Check sheet for the modelled part. Datum: model origin and axes. Units: mm. A direction names the side the tool comes from. Give positions to 0.01 mm unless a question says otherwise; leave off trailing zeros. Write each loop counter-clockwise with the first axis right and the second up, starting at its lowest first coordinate (ties: lowest second). Pieces come first, ordered by that corner, then holes. Notation, with made-up numbers: (36.5, 2) -> (43.5, 2) arc R16 ccw to (43.5, 12) -> close; hole circle Ø3 at (-26.5, 59). An arc over 180 degrees is marked (long way). Return JSON: item names as keys, results as strings.
from build123d import *
from build123d.topology import SkipClean

# Parameters (mm, degrees)
BASE_FLANGE1_DEPTH       = 2.54
SKETCHED_START           = 383.54
SKETCHED_BEND2_OUTLINE_W = 2.54
SKETCHED_BEND2_OUTLINE_H = 495.3
SKETCHED_BEND2_DEPTH     = 378.46
SKETCHED_START_2         = 381
SKETCHED_BEND2_2_DEPTH   = 2.221317884
SKETCHED_START_3         = 380.2634
SKETCHED_BEND2_3_DEPTH   = 3.2766
SKETCHED_START_4         = -438.15
SKETCHED_BEND2_4_DEPTH   = 495.3
SKETCHED_START_5         = 2.131240091
SKETCHED_BEND7_DEPTH     = 25
SKETCHED_BEND7_2_DEPTH   = 12.3
SKETCHED_START_6         = -384.2766
SKETCHED_BEND7_3_DEPTH   = 3.158240169
SKETCHED_START_7         = 0.118359831
SKETCHED_BEND7_4_DEPTH   = 3.158240169
SKETCHED_START_8         = 14.431240091
SKETCHED_BEND7_5_DEPTH   = 12.7
SKETCHED_BEND7_6_DEPTH   = 12.7
SKETCH20_R               = 8
CUT_EXTRUDE1_DEPTH       = 665.217598099
SKETCH21_R               = 12.7
CUT_EXTRUDE2_DEPTH       = 2.54
CUT_EXTRUDE3_DEPTH       = 2.54


with BuildPart() as part:
    # Base-Flange1: sheet metal written as solids
    # Sketch1 → Base-Flange1 (new body)
    with BuildSketch(Plane(origin=(0, 0, 0), x_dir=(1, 0, 0), z_dir=(0, 1, 0))):
        with BuildLine():
            Line((0, 0), (0, 381))
            Line((0, 381), (384.81, 381))
            Line((384.81, 381), (384.81, 438.15))
            Line((384.81, 438.15), (397.11, 438.15))
            ThreePointArc((397.11, 438.15), (406.090256121, 434.430256121), (409.81, 425.45))
            Line((409.81, 425.45), (409.81, 381))
            Line((409.81, 381), (690.157951031, 381))
            Line((690.157951031, 381), (762, 381))
            Line((762, 381), (762, 0.361010763))
            Line((762, 0.361010763), (690.158858088, 0))
            Line((690.158858088, 0), (409.81, 0))
            Line((409.81, 0), (409.81, -44.45))
            ThreePointArc((409.81, -44.45), (406.090256121, -53.430256121), (397.11, -57.15))
            Line((397.11, -57.15), (384.81, -57.15))
            Line((384.81, -57.15), (384.81, 0))
            Line((384.81, 0), (0, 0))
        make_face()
    extrude(amount=-BASE_FLANGE1_DEPTH)

    # Sketched Bend2: read off the stored shape, not the designer's step
    # Sketched Bend2 outline → Sketched Bend2 (cut)
    with BuildSketch(Plane.YZ.offset(SKETCHED_START)):
        with Locations((-1.27, -190.5)):
            Rectangle(SKETCHED_BEND2_OUTLINE_W, SKETCHED_BEND2_OUTLINE_H)
    extrude(amount=SKETCHED_BEND2_DEPTH, mode=Mode.SUBTRACT)

    # Sketched Bend2 2 outline → Sketched Bend2 2 (add)
    with BuildSketch(Plane.YZ.offset(SKETCHED_START_2)):
        with BuildLine():
            Line((2.131240091, 57.15), (2.131240091, 0))
            Line((2.131240091, 0), (0, 0))
            Line((0, 0), (0, -381))
            Line((0, -381), (2.131240091, -381))
            Line((2.131240091, -381), (2.131240091, -438.15))
            Line((2.131240091, -438.15), (14.431240091, -438.15))
            ThreePointArc((14.431240091, -438.15), (23.411496212, -434.430256121), (27.131240091, -425.45))
            Line((27.131240091, -425.45), (27.131240091, -381))
            Line((27.131240091, -381), (379.321240091, -381))
            Line((379.321240091, -381), (379.321240091, -0.361010763))
            Line((379.321240091, -0.361010763), (307.480098179, 0))
            Line((307.480098179, 0), (27.131240091, 0))
            Line((27.131240091, 0), (27.131240091, 44.45))
            ThreePointArc((27.131240091, 44.45), (23.411496212, 53.430256121), (14.431240091, 57.15))
            Line((14.431240091, 57.15), (2.131240091, 57.15))
        make_face()
    extrude(amount=SKETCHED_BEND2_2_DEPTH)

    # Sketched Bend2 3 outline → Sketched Bend2 3 (add)
    with BuildSketch(Plane.YZ.offset(SKETCHED_START_3)):
        with BuildLine():
            Line((2.131240091, 57.15), (2.131240091, 0))
            Line((2.131240091, 0), (0, 0))
            Line((0, 0), (0, -381))
            Line((0, -381), (2.131240091, -381))
            Line((2.131240091, -381), (2.131240091, -438.15))
            Line((2.131240091, -438.15), (14.431240091, -438.15))
            ThreePointArc((14.431240091, -438.15), (23.411496212, -434.430256121), (27.131240091, -425.45))
            Line((27.131240091, -425.45), (27.131240091, -381))
            Line((27.131240091, -381), (379.321240091, -381))
            Line((379.321240091, -381), (379.321240091, -0.361010763))
            Line((379.321240091, -0.361010763), (307.480098179, 0))
            Line((307.480098179, 0), (27.131240091, 0))
            Line((27.131240091, 0), (27.131240091, 44.45))
            ThreePointArc((27.131240091, 44.45), (23.411496212, 53.430256121), (14.431240091, 57.15))
            Line((14.431240091, 57.15), (2.131240091, 57.15))
        make_face()
    extrude(amount=SKETCHED_BEND2_3_DEPTH)

    # Sketched Bend2 4 outline → Sketched Bend2 4 (cut)
    with BuildSketch(Plane.XY.offset(SKETCHED_START_4)):
        with BuildLine():
            ThreePointArc((380.2634, 0), (380.784254855, 0.215745145), (381, 0.7366))
            Line((381, 0.7366), (381, 379.321240091))
            Line((381, 379.321240091), (380.2634, 379.321240091))
            Line((380.2634, 379.321240091), (380.2634, 0))
        make_face()
        with BuildLine():
            Line((383.54, -2.54), (383.54, 0.7366))
            ThreePointArc((383.54, 0.7366), (382.580306079, -1.580306079), (380.2634, -2.54))
            Line((380.2634, -2.54), (383.54, -2.54))
        make_face()
    extrude(amount=SKETCHED_BEND2_4_DEPTH, mode=Mode.SUBTRACT)

    # Sketched Bend7: read off the stored shape, not the designer's step
    # Sketched Bend7 outline → Sketched Bend7 (cut)
    with BuildSketch(Plane(origin=(0, 0, 0), x_dir=(1, 0, 0), z_dir=(0, 1, 0)).offset(SKETCHED_START_5)):
        with BuildLine():
            Line((383.54, -57.15), (383.54, 0))
            ThreePointArc((383.54, 0), (382.827542266, -2.039922057), (381, -3.192730493))
            Line((381, -3.192730493), (381, -57.15))
            Line((381, -57.15), (383.54, -57.15))
        make_face()
        with BuildLine():
            ThreePointArc((381, 384.192730493), (382.827542266, 383.039922057), (383.54, 381))
            Line((383.54, 381), (383.54, 438.15))
            Line((383.54, 438.15), (381, 438.15))
            Line((381, 438.15), (381, 384.192730493))
        make_face()
    extrude(amount=SKETCHED_BEND7_DEPTH, mode=Mode.SUBTRACT)

    # Sketched Bend7 2 outline → Sketched Bend7 2 (add)
    with BuildSketch(Plane(origin=(0, 0, 0), x_dir=(1, 0, 0), z_dir=(0, 1, 0)).offset(SKETCHED_START_5)):
        with BuildLine():
            ThreePointArc((380.2634, -3.2766), (380.634079664, -3.255565104), (381, -3.192730493))
            Line((381, -3.192730493), (381, 0))
            ThreePointArc((381, 0), (380.784254855, -0.520854855), (380.2634, -0.7366))
            Line((380.2634, -0.7366), (326.265359909, -0.7366))
            Line((326.265359909, -0.7366), (326.265359909, -3.2766))
            Line((326.265359909, -3.2766), (380.2634, -3.2766))
        make_face()
        with BuildLine():
            Line((381, 381), (381, 384.192730493))
            ThreePointArc((381, 384.192730493), (380.634079664, 384.255565104), (380.2634, 384.2766))
            Line((380.2634, 384.2766), (326.265359909, 384.2766))
            Line((326.265359909, 384.2766), (326.265359909, 381.7366))
            Line((326.265359909, 381.7366), (380.2634, 381.7366))
            ThreePointArc((380.2634, 381.7366), (380.784254855, 381.520854855), (381, 381))
        make_face()
    extrude(amount=SKETCHED_BEND7_2_DEPTH)

    # Sketched Bend7 3 outline → Sketched Bend7 3 (add)
    with BuildSketch(Plane.XY.offset(SKETCHED_START_6)):
        with BuildLine():
            Line((381, 14.431240091), (381, 27.131240091))
            Line((381, 27.131240091), (338.965359909, 27.131240091))
            ThreePointArc((338.965359909, 27.131240091), (329.985103788, 23.411496212), (326.265359909, 14.431240091))
            Line((326.265359909, 14.431240091), (381, 14.431240091))
        make_face()
    extrude(amount=SKETCHED_BEND7_3_DEPTH)

    # Sketched Bend7 4 outline → Sketched Bend7 4 (add)
    with BuildSketch(Plane.XY.offset(SKETCHED_START_7)):
        with BuildLine():
            Line((381, 14.431240091), (381, 27.131240091))
            Line((381, 27.131240091), (338.965359909, 27.131240091))
            ThreePointArc((338.965359909, 27.131240091), (329.985103788, 23.411496212), (326.265359909, 14.431240091))
            Line((326.265359909, 14.431240091), (381, 14.431240091))
        make_face()
    extrude(amount=SKETCHED_BEND7_4_DEPTH)

    # Sketched Bend7 5 outline → Sketched Bend7 5 (cut)
    with SkipClean():  # the faces are left unmerged after this step: merging them gives an invalid solid
        with BuildSketch(Plane(origin=(0, 0, 0), x_dir=(1, 0, 0), z_dir=(0, 1, 0)).offset(SKETCHED_START_8)):
            with BuildLine():
                Line((381, -3.2766), (381, -3.192730493))
                ThreePointArc((381, -3.192730493), (380.634079664, -3.255565104), (380.2634, -3.2766))
                Line((380.2634, -3.2766), (325, -3.276600014))
                Line((325, -3.276600014), (325, -5))
                Line((325, -5), (381.000000013, -5))
                Line((381.000000013, -5), (381, -3.2766))
            make_face()
            with BuildLine():
                ThreePointArc((380.2634, -0.7366), (380.740576963, -0.561143213), (380.990428549, -0.118359831))
                Line((380.990428549, -0.118359831), (325, -0.118359831))
                Line((325, -0.118359831), (325, -0.7366))
                Line((325, -0.7366), (380.2634, -0.7366))
            make_face()
            with BuildLine():
                Line((325, 381.118359831), (380.990428549, 381.118359831))
                ThreePointArc((380.990428549, 381.118359831), (380.740576963, 381.561143213), (380.2634, 381.7366))
                Line((380.2634, 381.7366), (325, 381.7366))
                Line((325, 381.7366), (325, 381.118359831))
            make_face()
            with BuildLine():
                ThreePointArc((380.2634, 384.2766), (380.634079664, 384.255565104), (381, 384.192730493))
                Line((381, 384.192730493), (381, 384.2766))
                Line((381, 384.2766), (381.000000039, 386))
                Line((381.000000039, 386), (325, 386))
                Line((325, 386), (325, 384.276600014))
                Line((325, 384.276600014), (380.2634, 384.2766))
            make_face()
        extrude(amount=SKETCHED_BEND7_5_DEPTH, mode=Mode.SUBTRACT)

    # Sketched Bend7 6 outline → Sketched Bend7 6 (add)
    with SkipClean():  # the faces are left unmerged after this step: merging them gives an invalid solid
        with BuildSketch(Plane(origin=(0, 0, 0), x_dir=(1, 0, 0), z_dir=(0, 1, 0)).offset(SKETCHED_START_8)):
            with BuildLine():
                Line((380.990428549, -0.118359831), (381, -0.118359831))
                Line((381, -0.118359831), (381, 0))
                ThreePointArc((381, 0), (380.997603238, -0.059373105), (380.990428549, -0.118359831))
            make_face()
            with BuildLine():
                ThreePointArc((380.990428549, 381.118359831), (380.997603238, 381.059373105), (381, 381))
                Line((381, 381), (381.000000039, 381.118359831))
                Line((381.000000039, 381.118359831), (380.990428549, 381.118359831))
            make_face()
        extrude(amount=SKETCHED_BEND7_6_DEPTH)

    # Sketch20 → Cut-Extrude1 (cut, through all)
    with SkipClean():  # the faces are left unmerged after this step: merging them gives an invalid solid
        with BuildSketch(Plane.XY.offset(3.2766)):
            with Locations((338.765359909, 14.631240091)):
                Circle(SKETCH20_R)
        extrude(amount=-CUT_EXTRUDE1_DEPTH, mode=Mode.SUBTRACT)

    # Sketch21 → Cut-Extrude2 (cut)
    with SkipClean():  # the faces are left unmerged after this step: merging them gives an invalid solid
        with BuildSketch(Plane(origin=(383.54, 0, 0), x_dir=(0, 0, -1), z_dir=(1, 0, 0))):
            with Locations(Location((190.5, 206.347240091, 0), (0, 0, 90))):
                Circle(SKETCH21_R)
        extrude(amount=-CUT_EXTRUDE2_DEPTH, mode=Mode.SUBTRACT)

    # Sketch22 → Cut-Extrude3 (cut)
    with SkipClean():  # the faces are left unmerged after this step: merging them gives an invalid solid
        with BuildSketch(Plane.XZ.offset(2.54)):
            with BuildLine():
                Line((101.704654894, -196.888541513), (152.504654894, -196.888541513))
                ThreePointArc((152.504654894, -196.888541513), (156.994782955, -198.748413452), (158.854654894, -203.238541513))
                Line((158.854654894, -203.238541513), (158.854654894, -254.038541513))
                ThreePointArc((158.854654894, -254.038541513), (156.994782955, -258.528669573), (152.504654894, -260.388541513))
                Line((152.504654894, -260.388541513), (101.704654894, -260.388541513))
                ThreePointArc((101.704654894, -260.388541513), (97.214526834, -258.528669573), (95.354654894, -254.038541513))
                Line((95.354654894, -254.038541513), (95.354654894, -203.238541513))
                ThreePointArc((95.354654894, -203.238541513), (97.214526834, -198.748413452), (101.704654894, -196.888541513))
            make_face()
        extrude(amount=-CUT_EXTRUDE3_DEPTH, mode=Mode.SUBTRACT)


solid = part.part
(1) Cross-section at C-C on z = -314.5. Enter the section's corners in (x, y), then the cut area to 3 significant figures.
Reply:
{"outline": "(0, -2.54) -> (380.26, -2.54) arc R3.28 ccw to (383.54, 0.74) -> (383.54, 379.32) -> (381, 379.32) -> (381, 0.74) arc R0.74 cw to (380.26, 0) -> (0, 0) -> close", "area": "1,940 mm^2"}
(2) Depth check by flat-ended pin: pin 1 Ø3.5 at (x, y) = (133, -0.5) entering from -Z; pin 2 Ø3 at (x, y) = (382, 166) entering from +Z; pin 3 Ø3 at (y, z) = (11, -383) entering from -X. Enter the tip coordinate at first touch or a pass-through.
Reply:
{"pin 1": "z = -381", "pin 2": "z = 0", "pin 3": "x = 326.27"}
(3) Cross-section at A-A on z = -190.5. Enter the section's corners in (x, y).
Reply:
{"outline": "(0, -2.54) -> (380.26, -2.54) arc R3.28 ccw to (383.54, 0.74) -> (383.54, 193.65) -> (381, 193.65) -> (381, 0.74) arc R0.74 cw to (380.26, 0) -> (0, 0) -> close; (381, 219.05) -> (383.54, 219.05) -> (383.54, 379.32) -> (381, 379.32) -> close"}
(4) Cross-section at D-D on z = -233.5. Enter the section's corners in (x, y), then the cut area to 3 significant figures.
Reply:
{"outline": "(0, -2.54) -> (95.35, -2.54) -> (95.35, 0) -> (0, 0) -> close; (158.85, -2.54) -> (380.26, -2.54) arc R3.28 ccw to (383.54, 0.74) -> (383.54, 379.32) -> (381, 379.32) -> (381, 0.74) arc R0.74 cw to (380.26, 0) -> (158.85, 0) -> close", "area": "1,770 mm^2"}
(5) Thickness scan on L1, parallel to X at y = 324.5, z = -80; L2, parallel to Y at x = 32.5, z = -292. Record the ranges inside material, lowest first.
Reply:
{"L1": "381 to 383.54", "L2": "-2.54 to 0"}
(6) Release check for a two-part mould opening along Z. For faces 1 (the cylindrical face through (382.29, 196.27, -198.23)), 2 (the flat face through (353, 15, -384.277)), 3 (the cylindrical face through (332.87, 20.04, -382.99)) record: pulls with the +Z half, pulls with the -Z half, needs draft (parallel to the pull), parting line crosses it, or undercut.
Reply:
{"face 1": "undercut", "face 2": "pulls with the -Z half", "face 3": "needs draft"}
(7) Cross-section at B-B on x = 132.5. Enter the section's corners in (y, z).
Reply:
{"outline": "(-2.54, -381) -> (0, -381) -> (0, -260.39) -> (-2.54, -260.39) -> close; (-2.54, -196.89) -> (0, -196.89) -> (0, 0) -> (-2.54, 0) -> close"}
(8) Set-up check for faces 4 (the flat face through (353, 14, -381.737)), 5 (the flat face through (193, 0, -193)), 6 (the flat face through (383.54, 187, -188)): record each of +Z, -Z, +X, -X, +Y, -Y from which the full face is reachable in a straight line by a thin tool's end or side.
Reply:
{"face 4": "-X, +Y, -Y", "face 5": "+Z, -Z, -X, +Y", "face 6": "+Z, -Z, +X, +Y, -Y"}
